Can you work these out from the drawing? Everything is in mm from the part's minimum corner. Coordinates: 2 decimals unless noted, no trailing zeros. Order: outer loops, then holes, each group sorted by start corner. A loop starts at its lowest first (then second) coordinate and runs counter-clockwise, first axis right, second up. Notation, with made-up numbers: (-5, 17.5) - (24, 17.5) arc R7 cw to (24, 30.5) - close; hole circle Ø11 at (4.5, 70). An arc over 180 degrees is marked (long way). Answer as CSV lines item,"result". Start each with the question number.
Item 1: I'm going to push a flat-ended pin straight in: pin 1 (12.5 mm diameter, centred on x = 90.01, y = 60.75, fed in from +Z). Where does the tip first touch, or does it pass through?
Item 2: Imagine slicing it at C-C on x = 92. List the corners of the cut face in (y, z) for me.
Item 3: Imagine slicing it at B-B on y = 94. Count the separate pieces of the cut face and the enclosed holes in it.
Item 4: Imagine slicing it at A-A on x = 17.5. List the corners of the cut face in (y, z) for me (1 decimal), and give its area (3 significant figures).
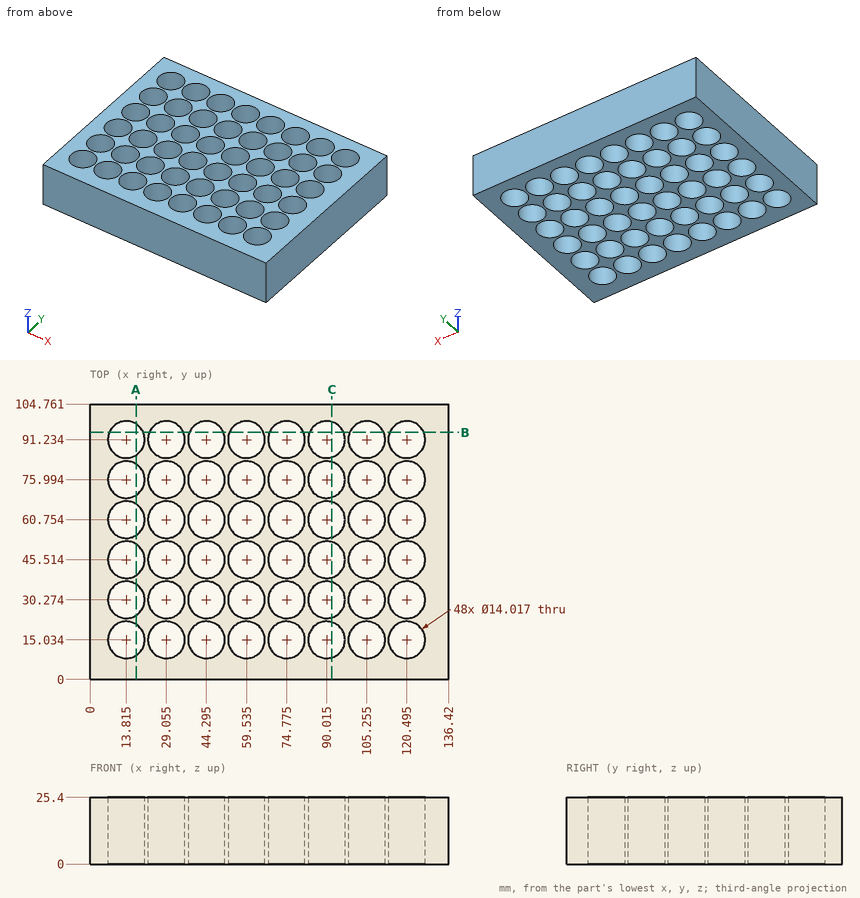
Responses:
1,pin 1,"passes through"
2,outline,"(0, 0) - (8.31, 0) - (8.31, 25.4) - (0, 25.4) - close; (21.76, 0) - (23.55, 0) - (23.55, 25.4) - (21.76, 25.4) - close; (37, 0) - (38.79, 0) - (38.79, 25.4) - (37, 25.4) - close; (52.24, 0) - (54.03, 0) - (54.03, 25.4) - (52.24, 25.4) - close; (67.48, 0) - (69.27, 0) - (69.27, 25.4) - (67.48, 25.4) - close; (82.72, 0) - (84.51, 0) - (84.51, 25.4) - (82.72, 25.4) - close; (97.96, 0) - (104.76, 0) - (104.76, 25.4) - (97.96, 25.4) - close"
3,separate pieces,"9"
3,enclosed holes,"0"
4,outline,"(0, 0) - (9.1, 0) - (9.1, 25.4) - (0, 25.4) - close; (21, 0) - (24.3, 0) - (24.3, 25.4) - (21, 25.4) - close; (36.2, 0) - (39.6, 0) - (39.6, 25.4) - (36.2, 25.4) - close; (51.5, 0) - (54.8, 0) - (54.8, 25.4) - (51.5, 25.4) - close; (66.7, 0) - (70, 0) - (70, 25.4) - (66.7, 25.4) - close; (82, 0) - (85.3, 0) - (85.3, 25.4) - (82, 25.4) - close; (97.2, 0) - (104.8, 0) - (104.8, 25.4) - (97.2, 25.4) - close"
4,area,"844 mm^2"
